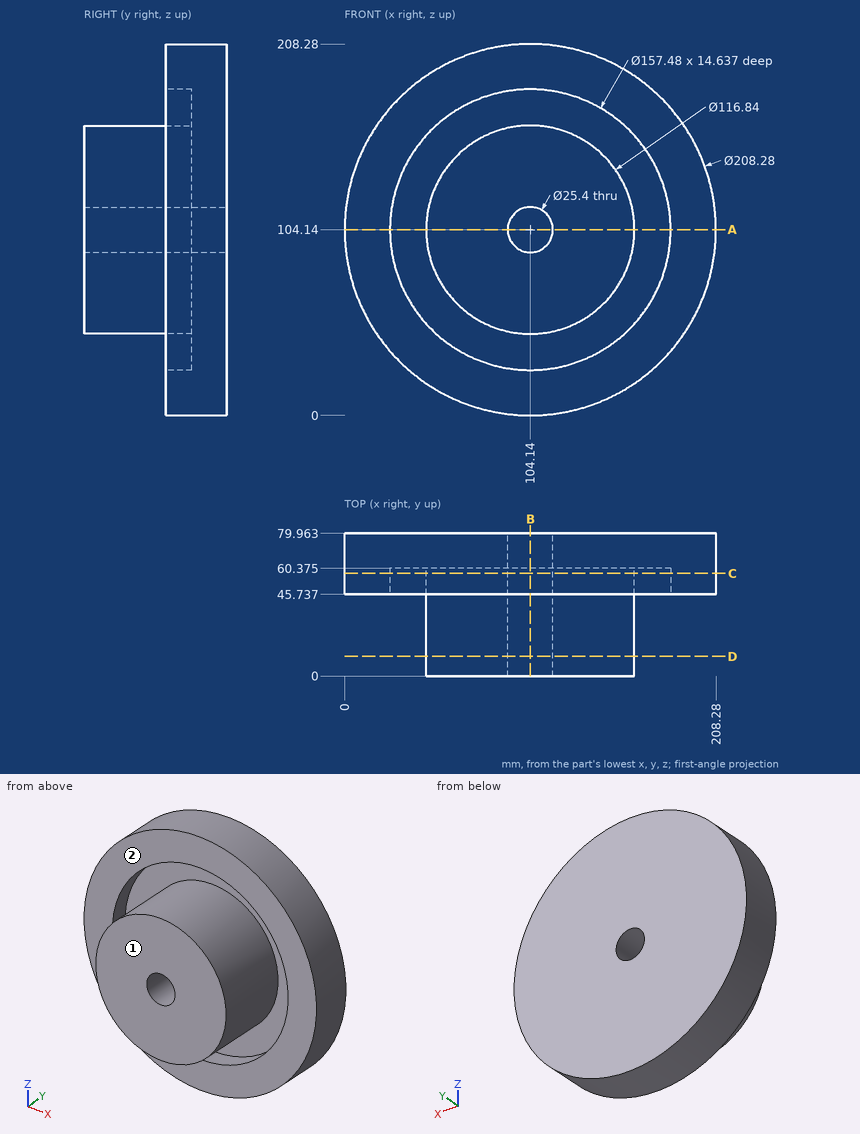
For this review, use the dimensioned drawing (mm, ordinates from the lowest corner) and the shaded views. A direction names the side the tool comes from. Coordinates: 2 decimals unless noted, no trailing zeros. Order: outer loops, then holes, each group sorted by start corner. A loop starts at its lowest first (then second) coordinate and runs counter-clockwise, first axis right, second up. Notation, with made-up numbers: (18, 17.25) - (58, 17.25) arc R30 ccw to (58, 45.25) - close; hole circle Ø6 at (14.5, 85.5). An arc over 180 degrees is marked (long way). Answer as a JSON object with one key per item and string values. Group by question number.
1. We need section B-B on x = 104.14. State the section outline as (y, z) points (1 decimal).
2. We need section D-D on y = 11. State the section outline as (x, z) points, then the cut area to 3 significant figures.
3. Clearance check with flat-ended pins moving along their axes: P1, Ø12, axis at y = 53.5, z = 179, coming from the -X side (1 decimal); P2, Ø5, axis at x = 47, y = 50, coming from the -Z side (1 decimal); P3, Ø5, axis at y = 48, z = 156, coming from the -X side. State where each tip first meets the part, or that it passes through.
4. For the marked faces 1 and 2, list the 3-axis set-ups (+Z, -Z, +X, -X, +Y, -Y) from which the entire face can be reached by the end or side of a thin tool; tool diameter is ignored.
5. We need section C-C on y = 57.5. State the section outline as (x, z) points.
6. For probe 1 along X at (y, z) = (57.5, 104.14); probe 2 along Z at (x, y) = (104, 22), list the stretches that pass through material, from the lowest coordinate up.
7. We need section A-A on z = 104.14. State the section outline as (x, y) points (1 decimal).
Final values:
{
 "1": {"outline": "(0, 45.7) - (60.4, 45.7) - (60.4, 25.4) - (45.7, 25.4) - (45.7, 0) - (80, 0) - (80, 91.4) - (0, 91.4) - close; (0, 116.8) - (80, 116.8) - (80, 208.3) - (45.7, 208.3) - (45.7, 182.9) - (60.4, 182.9) - (60.4, 162.6) - (0, 162.6) - close"},
 "2": {"outline": "circle Ø116.84 at (104.14, 104.14); hole circle Ø25.4 at (104.14, 104.14)", "area": "10,200 mm²"},
 "3": {"P1": "x = 26", "P2": "z = 15.5", "P3": "x = 12.44"},
 "4": {"face 1": "+Z, -Z, +X, -X, -Y", "face 2": "-Y"},
 "5": {"outline": "circle Ø208.28 at (104.14, 104.14); circle Ø116.84 at (104.14, 104.14); hole circle Ø157.48 at (104.14, 104.14); hole circle Ø25.4 at (104.14, 104.14)"},
 "6": {"probe 1": "0 to 25.4, 45.72 to 91.44, 116.84 to 162.56, 182.88 to 208.28", "probe 2": "45.72 to 91.44, 116.84 to 162.56"},
 "7": {"outline": "(0, 45.7) - (25.4, 45.7) - (25.4, 60.4) - (45.7, 60.4) - (45.7, 0) - (91.4, 0) - (91.4, 80) - (0, 80) - close; (116.8, 0) - (162.6, 0) - (162.6, 60.4) - (182.9, 60.4) - (182.9, 45.7) - (208.3, 45.7) - (208.3, 80) - (116.8, 80) - close"}
}
